Source: CAD feature listing. Evaluate the final solid. Frame: model axes, mm. A direction names the side the tool comes from. Round coordinates to 2 decimals unless told otherwise and drop trailing zeros. Loops run counter-clockwise (first coordinate to the right, second up) from the corner with the lowest first, then second, coordinate; pieces in that order, holes last.
(1) Section A-A, the plane y = 138.5. Return the cut outline in (x, z), plus the area to 3 significant figures.
(2) Set-up query: faces 4 (the flat face through (0, 18, 3)), 5 (the flat face through (3, 96.52, 3)), 6 (the flat face through (-127, 77, 3)), 7 (the flat face through (0, 236, 3)), 8 (the flat face through (-127, 18, 3)). Return all of +Z, -Z, +X, -X, +Y, -Y with unobstructed straight access to the full face (end or side cutting, diameter ignored); none if empty.
(3) Mould query, pull axis Y, two halves, no side actions, for faces 1 (the flat face through (3, 172.72, 3)), 2 (the flat face through (-130, 33.02, 3)), 3 (the flat face through (-133.35, 209, 3)). Classes: pulls with the +Y half, pulls with the -Y half, needs draft (parallel to the pull), parting line crosses it, or undercut.
(4) First-contact query: pin 1 Ø1 at (y, z) = (68.5, 2) entering from -X; pin 2 Ø1.9 at (x, z) = (-130, 3) entering from +Y; pin 3 Ø1.9 at (x, z) = (-131.5, 4) entering from -Y; pin 4 Ø10 at (x, y) = (-42.5, 93) entering from -Z. Flat tips, straight axial feed; report the tip coordinate or a pass-through.
(5) Material intervals for probe 1 along X at (y, z) = (75, 4), sorted ascending.
```python
from build123d import *

# Parameters (mm, degrees)
SKETCH1_W           = 139.7
SKETCH1_H           = 246.38
BOSS_EXTRUDE1_DEPTH = 6.35
SKETCH2_W           = 6.35
SKETCH2_H           = 26.67
SKETCH2_H_2         = 38.1
SKETCH2_H_3         = 25.4
SKETCH2_H_4         = 31.75
CUT_EXTRUDE1_DEPTH  = 6.35
SKETCH7_W           = 6.35
SKETCH7_H           = 26.67
SKETCH7_H_2         = 38.1
SKETCH7_H_3         = 25.4
CUT_EXTRUDE5_DEPTH  = 7.35
SKETCH8_W           = 127
SKETCH8_H           = 6.35
BOSS_EXTRUDE2_DEPTH = 3.81
SKETCH6_W           = 6.35
SKETCH6_H           = 1.27
CUT_EXTRUDE6_DEPTH  = 134.35


with BuildPart() as part:
    # Sketch1 → Boss-Extrude1 (new body)
    with BuildSketch(Plane.XY):
        with Locations((-63.5, 129.54)):
            Rectangle(SKETCH1_W, SKETCH1_H)
    extrude(amount=BOSS_EXTRUDE1_DEPTH)

    # Sketch2 → Cut-Extrude1 (cut)
    with BuildSketch(Plane(origin=(6.35, 0, 0), x_dir=(0, 0, -1), z_dir=(1, 0, 0))):
        with Locations((-3.175, 19.685)):
            Rectangle(SKETCH2_W, SKETCH2_H)
        with Locations((-3.175, 77.47)):
            Rectangle(SKETCH2_W, SKETCH2_H_2)
        with Locations((-3.175, 134.62)):
            Rectangle(SKETCH2_W, SKETCH2_H_3)
        with Locations((-3.175, 185.42)):
            Rectangle(SKETCH2_W, SKETCH2_H_3)
        with Locations((-3.175, 236.855)):
            Rectangle(SKETCH2_W, SKETCH2_H_4)
    extrude(amount=-CUT_EXTRUDE1_DEPTH, mode=Mode.SUBTRACT)

    # Sketch7 → Cut-Extrude5 (cut, through all)
    with BuildSketch(Plane(origin=(0, 0, 0), x_dir=(-1, 0, 0), z_dir=(0, 0, -1))):
        with Locations((130.175, 19.685)):
            Rectangle(SKETCH7_W, SKETCH7_H)
        with Locations((130.175, 77.47)):
            Rectangle(SKETCH7_W, SKETCH7_H_2)
        with Locations((130.175, 134.62)):
            Rectangle(SKETCH7_W, SKETCH7_H_3)
        with Locations((130.175, 185.42)):
            Rectangle(SKETCH7_W, SKETCH7_H_3)
        Polygon((127, 220.98), (133.35, 220.98), (133.35, 252.73), (127, 252.73), (127, 247.65), align=None)
    extrude(amount=-CUT_EXTRUDE5_DEPTH, mode=Mode.SUBTRACT)

    # Sketch8 → Boss-Extrude2 (add)
    with BuildSketch(Plane.XZ.offset(-6.35)):
        with Locations((-63.5, 3.175)):
            Rectangle(SKETCH8_W, SKETCH8_H)
    extrude(amount=BOSS_EXTRUDE2_DEPTH)

    # Sketch6 → Cut-Extrude6 (cut, through all)
    with BuildSketch(Plane(origin=(0, 0, 0), x_dir=(0, 0, -1), z_dir=(1, 0, 0))):
        with Locations((-3.175, 252.095)):
            Rectangle(SKETCH6_W, SKETCH6_H)
    extrude(amount=-CUT_EXTRUDE6_DEPTH, mode=Mode.SUBTRACT)


solid = part.part
```
Output values:
1. outline: (-127, 0) - (0, 0) - (0, 6.35) - (-127, 6.35) - close
1. area: 806 mm2
2. face 4: +Z, -Z, +X, -Y
2. face 5: +Z, -Z, +X
2. face 6: +Z, -Z, -X
2. face 7: +Z, -Z, +X, +Y
2. face 8: +Z, -Z, -X, -Y
3. face 1: undercut
3. face 2: pulls with the -Y half
3. face 3: needs draft
4. pin 1: stops at x = -127
4. pin 2: stops at y = 220.98
4. pin 3: stops at y = 33.02
4. pin 4: stops at z = 0
5. probe 1: x = -127 to 0
